Source: three-view drawing plus pictorial views. Frame: mm from the lowest corner of the part. A direction names the side the tool comes from. Round coordinates to 2 decimals unless told otherwise and drop trailing zeros. Loops run counter-clockwise (first coordinate to the right, second up) from the corner with the lowest first, then second, coordinate; pieces in that order, holes last. Notation, with made-up numbers: (42.25, 47) -> (64.25, 47) arc R14 cw to (64.25, 73) -> close; hole circle Ø11 at (-30, 5.5). An arc over 180 degrees is marked (long way). Answer in a Markdown table with one row per item.
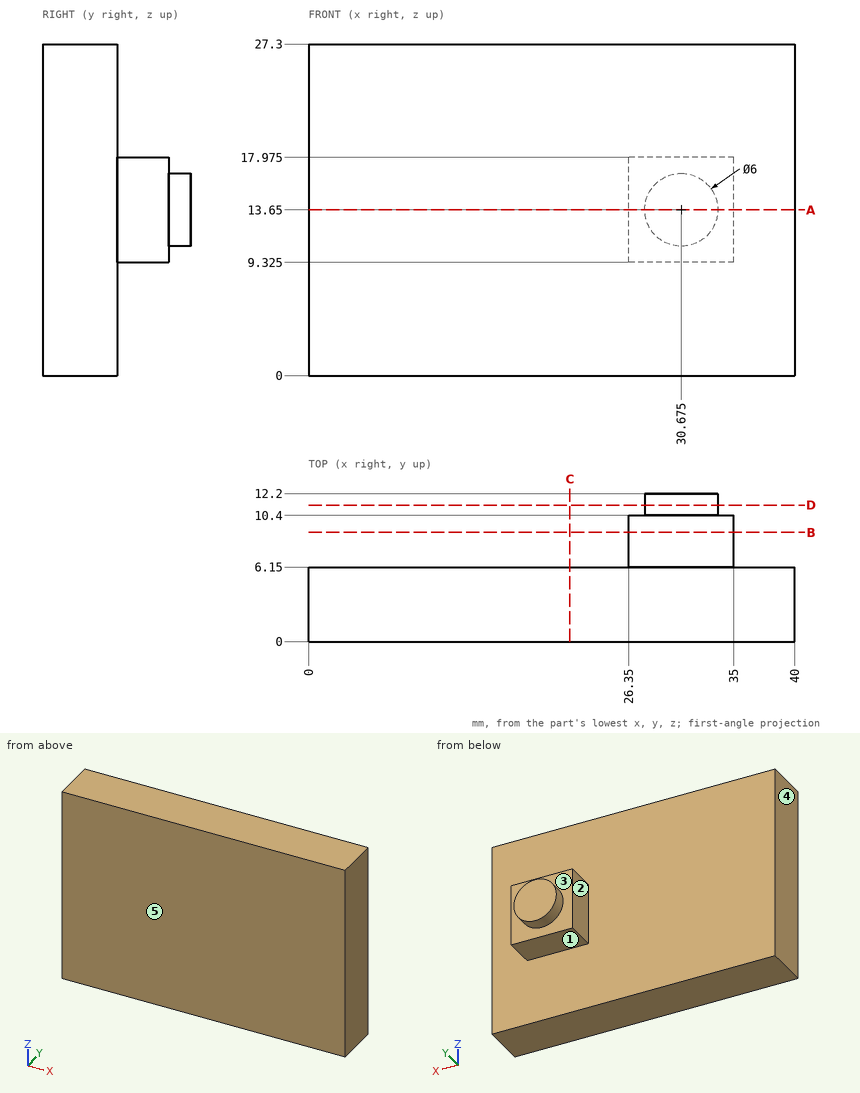
Item 1: Pin query (flat end, axial travel): pin 1 Ø1.3 at (x, y) = (31, 9.5) entering from +Z (3 decimals); pin 2 Ø8 at (x, z) = (10, 13) entering from +Y; pin 3 Ø1 at (x, z) = (29.5, 9) entering from +Y. Return the tip coordinate at first contact, or that it passes through.
Answer:
| item | result |
|---|---|
| pin 1 | stops at z = 17.975 |
| pin 2 | stops at y = 6.15 |
| pin 3 | stops at y = 10.4 |
Item 2: Cut plane D-D (y = 11.25). Output: boundary loops of the cut face in (x, z) (3 decimals), then the cut area to 3 significant figures.
Answer:
| item | result |
|---|---|
| outline | circle Ø6 at (30.675, 13.65) |
| area | 28.3 mm² |
Item 3: Cut plane A-A (z = 13.65). Output: boundary loops of the cut face in (x, y) (3 decimals).
Answer:
| item | result |
|---|---|
| outline | (0, 0) -> (40, 0) -> (40, 6.15) -> (35, 6.15) -> (35, 10.4) -> (33.675, 10.4) -> (33.675, 12.2) -> (27.675, 12.2) -> (27.675, 10.4) -> (26.35, 10.4) -> (26.35, 6.15) -> (0, 6.15) -> close |
Item 4: Cut plane C-C (x = 21.5). Output: boundary loops of the cut face in (y, z).
Answer:
| item | result |
|---|---|
| outline | (0, 0) -> (6.15, 0) -> (6.15, 27.3) -> (0, 27.3) -> close |
Item 5: Cut plane B-B (y = 9). Output: boundary loops of the cut face in (x, z) (3 decimals), then the cut area to 3 significant figures.
Answer:
| item | result |
|---|---|
| outline | (26.35, 9.325) -> (35, 9.325) -> (35, 17.975) -> (26.35, 17.975) -> close |
| area | 74.8 mm² |
Item 6: Line query: probe 1 along Y at (x, z) = (17, 7); probe 2 along Z at (x, y) = (32, 9) (3 decimals); probe 3 along Y at (x, z) = (33.5, 12.5). Output: solid intervals per line, ascending. Write a range as [from, to].
Answer:
| item | result |
|---|---|
| probe 1 | y = [0, 6.15] |
| probe 2 | z = [9.325, 17.975] |
| probe 3 | y = [0, 10.4] |
Item 7: Reachability of the marked faces 1, 2, 3, 4 and 5 from +Z, -Z, +X, -X, +Y, -Y: full face, straight path, thin tool, end or side. Return the list, or none.
Answer:
| item | result |
|---|---|
| face 1 | -Z, +X, -X, +Y |
| face 2 | +Z, -Z, -X, +Y |
| face 3 | +Y |
| face 4 | +Z, -Z, -X, +Y, -Y |
| face 5 | +Z, -Z, +X, -X, -Y |
